from build123d import *

# Parameters (mm, degrees)
SKETCH1_W           = 30
SKETCH1_H           = 20
BOSS_EXTRUDE1_DEPTH = 4
CUT_EXTRUDE1_DEPTH  = 37.276714294
SKETCH3_W           = 30
SKETCH3_H           = 17
BOSS_EXTRUDE2_DEPTH = 1
SKETCH4_R           = 4.1
CUT_EXTRUDE2_DEPTH  = 37.400549446


with BuildPart() as part:
    # Sketch1 → Boss-Extrude1 (new body)
    with BuildSketch(Plane(origin=(0, 0, 0), x_dir=(0, 0, -1), z_dir=(1, 0, 0))):
        with Locations((15, 10)):
            Rectangle(SKETCH1_W, SKETCH1_H)
    extrude(amount=BOSS_EXTRUDE1_DEPTH)

    # Sketch2 → Cut-Extrude1 (cut, through all)
    with BuildSketch(Plane(origin=(4, 0, 0), x_dir=(0, 0, -1), z_dir=(1, 0, 0))):
        with BuildLine():
            Line((4.205771366, 16), (19.205771366, 41.980762114))
            Line((19.205771366, 41.980762114), (34.794228634, 32.980762114))
            Line((34.794228634, 32.980762114), (19.794228634, 7))
            ThreePointArc((19.794228634, 7), (7.5, 3.705771366), (4.205771366, 16))
        make_face()
    extrude(amount=-CUT_EXTRUDE1_DEPTH, mode=Mode.SUBTRACT)

    # Sketch3 → Boss-Extrude2 (add)
    with BuildSketch(Plane(origin=(4, 0, 0), x_dir=(0, 0, -1), z_dir=(1, 0, 0))):
        with Locations((15, 8.5)):
            Rectangle(SKETCH3_W, SKETCH3_H)
    extrude(amount=BOSS_EXTRUDE2_DEPTH)

    # Sketch4 → Cut-Extrude2 (cut, through all)
    with BuildSketch(Plane(origin=(5, 0, 0), x_dir=(0, 0, -1), z_dir=(1, 0, 0))):
        with Locations((12.5, 12.366025404)):
            Circle(SKETCH4_R)
    extrude(amount=-CUT_EXTRUDE2_DEPTH, mode=Mode.SUBTRACT)


solid = part.part
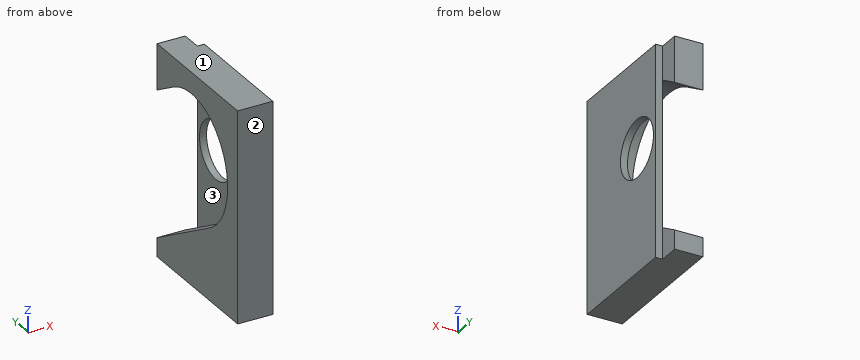
Build history of the part. All positions in model axes, mm. Face numbers are marked on the shaded views. Round coordinates to 2 decimals unless told otherwise and drop trailing zeros. Order: outer loops, then holes, each group sorted by start corner. A loop starts at its lowest first (then second) coordinate and runs counter-clockwise, first axis right, second up. Notation, with made-up numbers: M 10,51 L 46,51 A32 cw 46,86 Z; hole C 33.5,9 d9. An arc over 180 degrees is marked long. Use CSV: the item, a comma, the result in double quotes. Start each with the question number.
(1) Cut at D-D on z = -1.75. List the corners of the cut face in (x, y).
(2) Cut at B-B on y = 11.5. List the corners of the cut face in (x, z).
(3) Flat gauge pins, fed straight in: P1, Ø1.5, axis at x = 1.5, z = -22, coming from the +Y side; P2, Ø0.9, axis at y = 19, z = -3.5, coming from the +X side; P3, Ø3, axis at x = 0.5, y = 16, coming from the +Z side. Where does each tip first touch, or does it go through?
(4) Mould opens along Z. For the marked faces 1, 2 and 3 say: +Z half, -Z half, draft (parallel to the pull), parting line (faces both ways), or undercut.
(5) Drill centre lines: probe 1 along Y at (x, z) = (4.7, -12.5); probe 2 along X at (y, z) = (18.25, -3.75); probe 3 along X at (y, z) = (5, -15.5). Where is each one in solid material? Low to high.
(6) Cut at A-A on z = -12. List the corners of the cut face in (x, y), then the cut area to 3 significant figures.
Findings:
1,outline,"M 0,0 L 5,0 L 5,17 L 4,17 L 4,20 L 0,20 Z"
2,outline,"M 0,-30 L 5,-30 L 5,-16.51 L 4,-16.51 L 4,-22.39 L 0,-22.39 Z; M 0,-3 L 4,-3 L 4,-8.49 L 5,-8.49 L 5,0 L 0,0 Z"
3,P1,"stops at y = 12.12"
3,P2,"stops at x = 4"
3,P3,"stops at z = 0"
4,face 1,"+Z half"
4,face 2,"draft"
4,face 3,"undercut"
5,probe 1,"y = 0 to 8.27, 16.47 to 17"
5,probe 2,"x = 0 to 4"
5,probe 3,"x = 4 to 5"
6,outline,"M 0,0 L 5,0 L 5,8.3 L 4,8.3 L 4,2.5 L 0,2.5 Z; M 4,16.44 L 5,16.44 L 5,17 L 4,17 Z"
6,area,"18.9 mm^2"
